Check sheet for the modelled part. Datum: model origin and axes. Units: mm. Round coordinates to 2 decimals unless told otherwise and drop trailing zeros. Write each loop counter-clockwise with the first axis right and the second up, starting at its lowest first coordinate (ties: lowest second). Pieces come first, ordered by that corner, then holes. Notation, with made-up numbers: M 24.25,45.25 L 62.25,45.25 A23 ccw 62.25,72.25 Z; hole C 21.25,10.5 d3. An arc over 180 degrees is marked long. Answer in a Markdown table with one row per item.
```python
from build123d import *

# Parameters (mm, degrees)
BOSS_EXTRUDE1_DEPTH = 3.175
SKETCH2_R           = 2.5527
CUT_EXTRUDE1_DEPTH  = 136.04018152
SKETCH3_R           = 2.5527
CUT_EXTRUDE2_DEPTH  = 136.04018152


with BuildPart() as part:
    # Sketch1 → Boss-Extrude1 (new body)
    with BuildSketch(Plane(origin=(0, 0, 0), x_dir=(1, 0, 0), z_dir=(0, 1, 0))):
        Polygon((0, 0), (50.8, 0), (50.8, 76.2), (88.9, 76.2), (88.9, 101.6), (-38.1, 101.6), (-38.1, 76.2), (0, 76.2), align=None)
    extrude(amount=BOSS_EXTRUDE1_DEPTH)

    # Sketch2 → Cut-Extrude1 (cut, through all)
    with BuildSketch(Plane(origin=(0, 3.175, 0), x_dir=(1, 0, 0), z_dir=(0, 1, 0))):
        with Locations(Location((38.1, 6.35, 0), (0, 0, 270))):
            Circle(SKETCH2_R)
        with Locations(Location((12.7, 6.35, 0), (0, 0, 270))):
            Circle(SKETCH2_R)
        with Locations(Location((38.1, 19.05, 0), (0, 0, 270))):
            Circle(SKETCH2_R)
        with Locations(Location((12.7, 19.05, 0), (0, 0, 270))):
            Circle(SKETCH2_R)
        with Locations(Location((38.1, 31.75, 0), (0, 0, 270))):
            Circle(SKETCH2_R)
        with Locations(Location((12.7, 31.75, 0), (0, 0, 270))):
            Circle(SKETCH2_R)
        with Locations(Location((38.1, 44.45, 0), (0, 0, 270))):
            Circle(SKETCH2_R)
        with Locations(Location((12.7, 44.45, 0), (0, 0, 270))):
            Circle(SKETCH2_R)
        with Locations(Location((38.1, 57.15, 0), (0, 0, 270))):
            Circle(SKETCH2_R)
        with Locations(Location((12.7, 57.15, 0), (0, 0, 270))):
            Circle(SKETCH2_R)
        with Locations(Location((38.1, 69.85, 0), (0, 0, 270))):
            Circle(SKETCH2_R)
        with Locations(Location((12.7, 69.85, 0), (0, 0, 270))):
            Circle(SKETCH2_R)
    extrude(amount=-CUT_EXTRUDE1_DEPTH, mode=Mode.SUBTRACT)

    # Sketch3 → Cut-Extrude2 (cut, through all)
    with BuildSketch(Plane(origin=(0, 3.175, 0), x_dir=(1, 0, 0), z_dir=(0, 1, 0))):
        with Locations(Location((76.2, 88.9, 0), (0, 0, 270))):
            Circle(SKETCH3_R)
        with Locations(Location((63.5, 88.9, 0), (0, 0, 270))):
            Circle(SKETCH3_R)
        with Locations(Location((50.8, 88.9, 0), (0, 0, 270))):
            Circle(SKETCH3_R)
        with Locations(Location((38.1, 88.9, 0), (0, 0, 270))):
            Circle(SKETCH3_R)
        with Locations(Location((25.4, 88.9, 0), (0, 0, 270))):
            Circle(SKETCH3_R)
        with Locations(Location((12.7, 88.9, 0), (0, 0, 270))):
            Circle(SKETCH3_R)
        with Locations(Location((0, 88.9, 0), (0, 0, 270))):
            Circle(SKETCH3_R)
        with Locations(Location((-12.7, 88.9, 0), (0, 0, 270))):
            Circle(SKETCH3_R)
        with Locations(Location((-25.4, 88.9, 0), (0, 0, 270))):
            Circle(SKETCH3_R)
    extrude(amount=-CUT_EXTRUDE2_DEPTH, mode=Mode.SUBTRACT)


solid = part.part
```
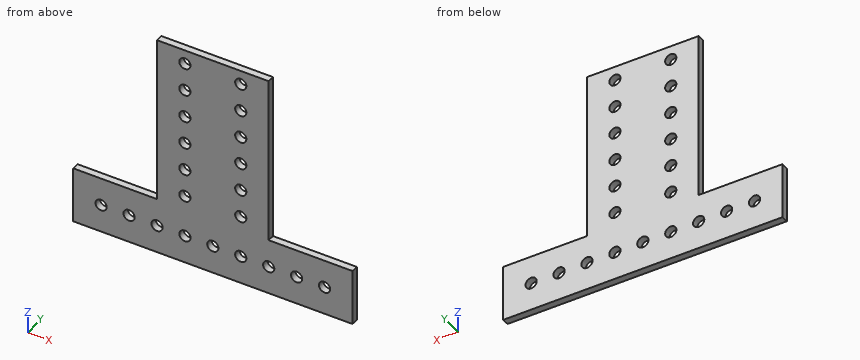
1. Section check B-B, the plane z = -69.85. Record the cut outline in (x, y) (3 decimals).
Found:
| item | result |
|---|---|
| outline | M 0,0 L 10.147,0 L 10.147,3.175 L 0,3.175 Z; M 15.253,0 L 35.547,0 L 35.547,3.175 L 15.253,3.175 Z; M 40.653,0 L 50.8,0 L 50.8,3.175 L 40.653,3.175 Z |
2. Section check C-C, the plane y = 1.95. Count the separate pieces of the cut face and the enclosed holes in it, and give its area (3 significant figures).
Found:
| item | result |
|---|---|
| separate pieces | 1 |
| enclosed holes | 21 |
| area | 6,670 mm2 |
3. Section check D-D, the plane x = 25.4. Record the cut outline in (y, z) (3 decimals), and give its area (3 significant figures).
Found:
| item | result |
|---|---|
| outline | M 0,-101.6 L 3.175,-101.6 L 3.175,-91.453 L 0,-91.453 Z; M 0,-86.347 L 3.175,-86.347 L 3.175,0 L 0,0 Z |
| area | 306 mm2 |
4. Section check A-A, the plane x = 76.2. Record the cut outline in (y, z) (3 decimals), and give its area (3 significant figures).
Found:
| item | result |
|---|---|
| outline | M 0,-101.6 L 3.175,-101.6 L 3.175,-91.453 L 0,-91.453 Z; M 0,-86.347 L 3.175,-86.347 L 3.175,-76.2 L 0,-76.2 Z |
| area | 64.4 mm2 |
5. Go/stop test with a flat-tipped pin: pin 1 (1 mm diameter, centred on y = 1, z = -53.5, fed in from -X). Record where the tip stops, or that it passes through.
Found:
| item | result |
|---|---|
| pin 1 | stops at x = 0 |
6. Scan lines: L1, parallel to X at y = 2.25, z = -6.35; L2, parallel to Z at x = -12.5, y = 2.7; L3, parallel to X at y = 0.4, z = -45. Record each from-to range of solid material in increasing order.
Found:
| item | result |
|---|---|
| L1 | x = 0 to 10.15, 15.25 to 35.55, 40.65 to 50.8 |
| L2 | z = -101.6 to -91.44, -86.36 to -76.2 |
| L3 | x = 0 to 10.21, 15.19 to 35.61, 40.59 to 50.8 |
